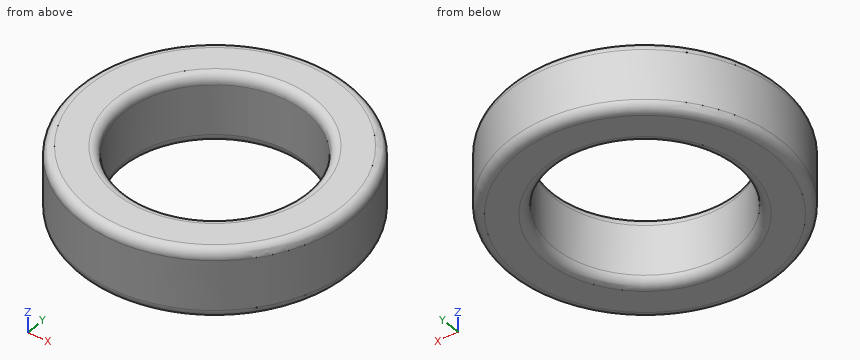
from build123d import *

# Parameters (mm, degrees)
SKETCH2_R           = 7.62
SKETCH2_R_2         = 5.08
BOSS_EXTRUDE1_DEPTH = 3.81
FILLET1_R           = 0.508
FILLET2_R           = 0.508
FILLET3_R           = 0.508
FILLET4_R           = 0.508


with BuildPart() as part:
    # Sketch2 → Boss-Extrude1 (new body)
    with BuildSketch(Plane.XY):
        with Locations(Location((0, 0, 0), (0, 0, 180))):
            Circle(SKETCH2_R)
        with Locations(Location((0, 0, 0), (0, 0, 180))):
            Circle(SKETCH2_R_2, mode=Mode.SUBTRACT)
    extrude(amount=BOSS_EXTRUDE1_DEPTH)

    # Fillet1
    fillet1_edges = [part.edges().sort_by_distance(p)[0] for p in [
        (5.08, 0, 3.81),
    ]]
    fillet(fillet1_edges, radius=FILLET1_R)

    # Fillet2
    fillet2_edges = [part.edges().sort_by_distance(p)[0] for p in [
        (5.08, 0, 0),
    ]]
    fillet(fillet2_edges, radius=FILLET2_R)

    # Fillet3
    fillet3_edges = [part.edges().sort_by_distance(p)[0] for p in [
        (7.62, 0, 0),
    ]]
    fillet(fillet3_edges, radius=FILLET3_R)

    # Fillet4
    fillet4_edges = [part.edges().sort_by_distance(p)[0] for p in [
        (7.62, 0, 3.81),
    ]]
    fillet(fillet4_edges, radius=FILLET4_R)


solid = part.part
Input: part model. Units: mm. Frame: model coordinates. Give positions to 0.01 mm unless a question says otherwise; leave off trailing zeros. Write each loop counter-clockwise with the first axis right and the second up, starting at its lowest first coordinate (ties: lowest second). Pieces come first, ordered by that corner, then holes. Notation, with made-up numbers: M 84.5,66 L 135.5,66 A24 cw 135.5,92 Z; hole C 14,30.5 d6. An arc over 180 degrees is marked long. Use one line per item in the form item = value.
1. Cut plane C-C on z = 2.1. Return loops of the section in (x, y).
Outcome:
outline = C 0,0 d15.24; hole C 0,0 d10.16
2. Cut plane A-A on y = 0. Return loops of the section in (x, z), and give its area (3 significant figures).
Outcome:
outline = M -7.62,0.51 A0.51 ccw -7.11,0 L -5.59,0 A0.51 ccw -5.08,0.51 L -5.08,3.3 A0.51 ccw -5.59,3.81 L -7.11,3.81 A0.51 ccw -7.62,3.3 Z; M 5.08,0.51 A0.51 ccw 5.59,0 L 7.11,0 A0.51 ccw 7.62,0.51 L 7.62,3.3 A0.51 ccw 7.11,3.81 L 5.59,3.81 A0.51 ccw 5.08,3.3 Z
area = 18.9 mm²
3. Ray query, L1, parallel to Y at x = 0, z = 1.85; L2, parallel to X at y = -2, z = 2.3; L3, parallel to Y at x = 1.25, z = 3.55. Return the intervals inside material, ascending.
Outcome:
L1 = -7.62 to -5.08, 5.08 to 7.62
L2 = -7.35 to -4.67, 4.67 to 7.35
L3 = -7.45 to -4.99, 4.99 to 7.45
4. Cut plane D-D on z = 3.6. Return loops of the section in (x, y).
Outcome:
outline = C 0,0 d15.05; hole C 0,0 d10.35
5. First-contact query: P1, Ø1.5, axis at x = -3, y = -0.5, coming from the -Z side; P2, Ø1, axis at y = 5, z = 1, coming from the +X side; P3, Ø1, axis at x = -1.5, z = 1.5, coming from the -Y side; P4, Ø1, axis at x = 4.5, z = 0.5, coming from the +Y side. Flat tips, straight axial feed; report the tip coordinate or a pass-through.
Outcome:
P1 = through
P2 = 6.15
P3 = -7.55
P4 = 6.49
